Design review of the part shown in the three views and the two pictorial views. Dimensions are in mm from the part's minimum x, y and z. A direction names the side the tool comes from. Give positions to 0.01 mm unless a question says otherwise; leave off trailing zeros. Loops run counter-clockwise (first coordinate to the right, second up) from the corner with the lowest first, then second, coordinate; pieces in that order, holes last. Notation, with made-up numbers: (14, 12.5) - (33, 12.5) arc R16 ccw to (33, 38.5) - close; hole circle Ø6 at (35, 51.25). An arc over 180 degrees is marked (long way). Answer as a JSON object with one key per item and string values.
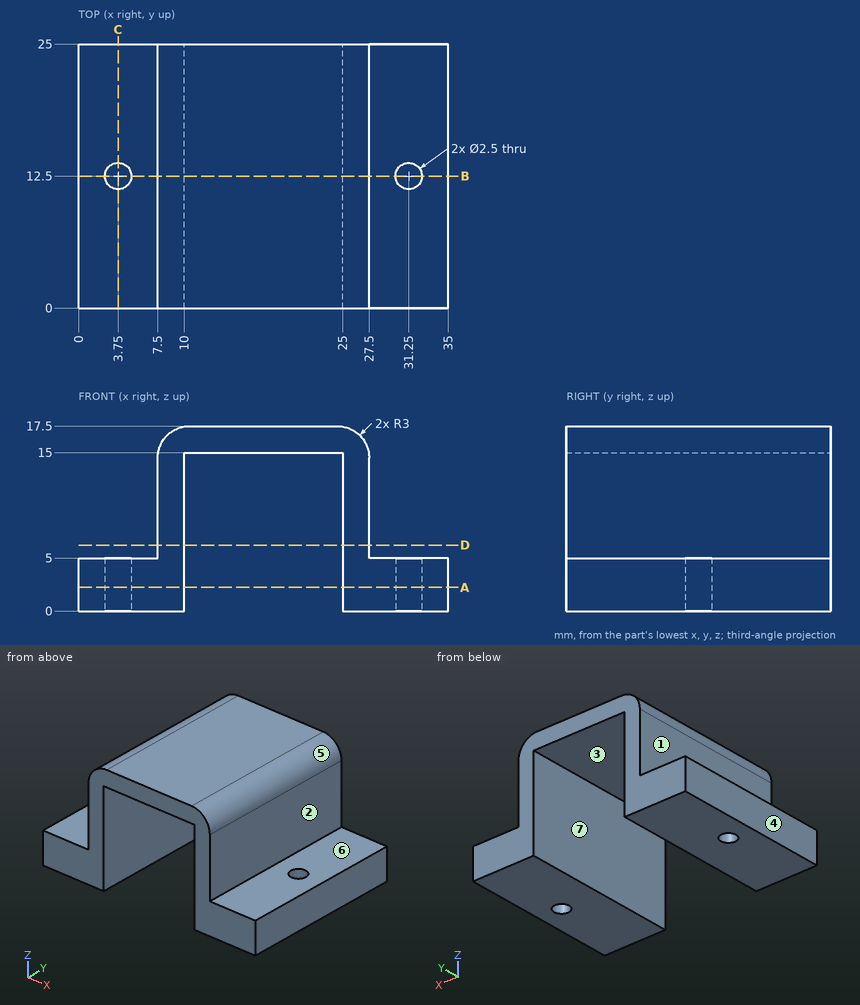
Q1. Consider section A-A, the plane z = 2.25. State the section outline as (x, y) points.
Results:
{"outline": "(0, 0) - (10, 0) - (10, 25) - (0, 25) - close; (25, 0) - (35, 0) - (35, 25) - (25, 25) - close; hole circle Ø2.5 at (3.75, 12.5); hole circle Ø2.5 at (31.25, 12.5)"}
Q2. Clearance check with flat-ended pins moving along their axes: pin 1 Ø6 at (x, y) = (32.5, 11.5) entering from +Z; pin 2 Ø10 at (x, y) = (31, 21.5) entering from +Z; pin 3 Ø3 at (y, z) = (13.5, 10.5) entering from -X. State where each tip first meets the part, or that it passes through.
Results:
{"pin 1": "stops at z = 5", "pin 2": "stops at z = 17.1", "pin 3": "stops at x = 7.5"}
Q3. Consider section D-D, the plane z = 6.25. State the section outline as (x, y) points, plus the area to 3 significant figures.
Results:
{"outline": "(7.5, 0) - (10, 0) - (10, 25) - (7.5, 25) - close; (25, 0) - (27.5, 0) - (27.5, 25) - (25, 25) - close", "area": "125 mm^2"}
Q4. To check wall thickness, follow probe 1 along X at (y, z) = (12.5, 3.25); probe 2 along X at (y, z) = (16.5, 12); probe 3 along Y at (x, z) = (3.75, 1.75). State the ranges of each line that lie inside material, in increasing order. Write a range as [from, to].
Results:
{"probe 1": "x = [0, 2.5], [5, 10], [25, 30], [32.5, 35]", "probe 2": "x = [7.5, 10], [25, 27.5]", "probe 3": "y = [0, 11.25], [13.75, 25]"}
Q5. Consider section B-B, the plane y = 12.5. State the section outline as (x, z) points, plus the area to 3 significant figures.
Results:
{"outline": "(0, 0) - (2.5, 0) - (2.5, 5) - (0, 5) - close; (5, 0) - (10, 0) - (10, 15) - (25, 15) - (25, 0) - (30, 0) - (30, 5) - (27.5, 5) - (27.5, 14.5) arc R3 ccw to (24.5, 17.5) - (10.5, 17.5) arc R3 ccw to (7.5, 14.5) - (7.5, 5) - (5, 5) - close; (32.5, 0) - (35, 0) - (35, 5) - (32.5, 5) - close", "area": "171 mm^2"}
Q6. For the marked faces 1, 2 and 3, list the 3-axis set-ups (+Z, -Z, +X, -X, +Y, -Y) from which the entire face can be reached by the end or side of a thin tool; tool diameter is ignored.
Results:
{"face 1": "+Z, -X, +Y, -Y", "face 2": "+Z, +X, +Y, -Y", "face 3": "-Z, +Y, -Y"}
Q7. Consider section C-C, the plane x = 3.75. State the section outline as (y, z) points, plus the area to 4 significant figures.
Results:
{"outline": "(0, 0) - (11.25, 0) - (11.25, 5) - (0, 5) - close; (13.75, 0) - (25, 0) - (25, 5) - (13.75, 5) - close", "area": "112.5 mm^2"}
Q8. The part is to be moulded in two halves that separate along X. For the marked faces 4, 5, 6 and 7, say which applies: +X half, -X half, draft (parallel to the pull), parting line (faces both ways), or undercut.
Results:
{"face 4": "-X half", "face 5": "+X half", "face 6": "draft", "face 7": "undercut"}
